from build123d import *

# Parameters (mm, degrees)
F0_W      = 1200
F0_H      = 2200
F1_DEPTH  = 40
F2_W      = 50
F2_H      = 1000
F3_DEPTH  = 10
F5_DEPTH  = 40.001
F6_R      = 25
F8_DEPTH  = 40.001
F9_W      = 25
F9_H      = 50
F10_DEPTH = 40.001
F12_D     = 14
F12_DEPTH = 31
F12_TIP   = 4.2060243332


with BuildPart() as f1:
    # F0 (on Front) → F1 (new body)
    with BuildSketch(Plane.XZ):
        Rectangle(F0_W, F0_H)
    extrude(amount=F1_DEPTH)

    # F2 (on face) → F3 (cut)
    with BuildSketch(Plane(origin=(0, 0, 0), x_dir=(-1, 0, 0), z_dir=(0, 1, 0))):
        with Locations((525, -600)):
            Rectangle(F2_W, F2_H)
    extrude(amount=-F3_DEPTH, mode=Mode.SUBTRACT)

    # F4 (on face) → F5 (cut, through all)
    with BuildSketch(Plane.XZ.offset(40)):
        with BuildLine():
            Line((-600, 300), (-600, 0))
            Line((-600, 0), (-350, 0))
            ThreePointArc((-350, 0), (-279.2893218813, 29.2893218813), (-250, 100))
            ThreePointArc((-250, 100), (-308.5786437627, 241.4213562373), (-450, 300))
            Line((-450, 300), (-600, 300))
        make_face()
    extrude(amount=-F5_DEPTH, mode=Mode.SUBTRACT)

    # F6
    f6_edges = [f1.edges().sort_by_distance(p)[0] for p in [
        (-600, -20, 300),
        (-600, -20, 0),
    ]]
    fillet(f6_edges, radius=F6_R)

    # F7 (on face) → F8 (cut, through all)
    with BuildSketch(Plane.XZ.offset(40)):
        with BuildLine():
            Line((-549.1, 1100), (-600, 1100))
            Line((-600, 1100), (-600, 325))
            ThreePointArc((-600, 325), (-592.6776695297, 307.3223304703), (-575, 300))
            Line((-575, 300), (-549.1, 300))
            Line((-549.1, 300), (-549.1, 1100))
        make_face()
    extrude(amount=-F8_DEPTH, mode=Mode.SUBTRACT)

    # F9 (on face) → F10 (cut, through all)
    with BuildSketch(Plane.XZ.offset(40)):
        with Locations((-587.5, -325)):
            Rectangle(F9_W, F9_H)
        with Locations((-587.5, -775)):
            Rectangle(F9_W, F9_H)
    extrude(amount=-F10_DEPTH, mode=Mode.SUBTRACT)

    # F12
    with Locations(Plane(origin=(-600, 0, 0), x_dir=(0, -1, 0), z_dir=(-1, 0, 0))):
        with Locations((20, -1050), (20, -950), (20, -850), (20, -700), (20, -600), (20, -500), (20, -400), (20, -250), (20, -150), (20, -50)):
            Hole(F12_D / 2, depth=F12_DEPTH)
            with Locations((0, 0, -(F12_DEPTH + F12_TIP / 2))):  # 118° drill point
                Cone(0, F12_D / 2, F12_TIP, mode=Mode.SUBTRACT)


solid = f1.part
Source: CAD feature listing. Evaluate the final solid. Frame: model axes, mm. A direction names the side the tool comes from. Give positions to 0.01 mm unless a question says otherwise; leave off trailing zeros. Loops run counter-clockwise (first coordinate to the right, second up) from the corner with the lowest first, then second, coordinate; pieces in that order, holes last. Notation, with made-up numbers: (67.5, 45) -> (96.5, 45) arc R27 cw to (96.5, 61) -> close; hole circle Ø8 at (24, -36.5). An arc over 180 degrees is marked (long way). Use a Markdown table: item, result. Add a question column.
1) Reachability of faces 4 (the face through (-464, -20, 0)), 5 (the face through (-8, -20, -1100)), 6 (the face through (-525, -10, -593)), 7 (the face through (-600, -20, -164)), 8 (the face through (-549.1, -20, 694)) from +Z, -Z, +X, -X, +Y, -Y: full face, straight path, thin tool, end or side. Return the list, or none.
2) Section query C-C, the plane z = 250. Return the cut outline in (x, y), then the cut area to 3 significant figures.
3) Section query B-B, the plane z = 588. Return the cut outline in (x, y).
4) Line query: line 1 along X through (y, z) = (-5, -876.5); line 2 along Y through (x, z) = (-581.5, -50); line 3 along X through (y, z) = (-3, 671). Output: solid intervals per line, ascending. Write a range as [from, to].
5) Pull-direction query (Z, two-part tool) for faces 1 (the face through (-600, -20, -553)), 2 (the face through (-575, -20, -325)), 3 (the face through (17, -20, 1100)); classes: +Z half, -Z half, draft (parallel to the pull), parting line (faces both ways), or undercut.
6) First-contact query: pin 1 (11 mm diameter, centred on y = -20, z = -700, fed in from -X); pin 2 (2 mm diameter, centred on y = -35, z = 664, fed in from -X); pin 3 (3 mm diameter, centred on x = -525, y = -5.5, fed in from -Z); pin 4 (18 mm diameter, centred on y = -20, z = -500, fed in from -X). Flat tips, straight axial feed; report the tip coordinate or a pass-through.
7) Section query A-A, the plane x = -321. Return the cut outline in (y, z).
Numbers:
| question | item | result |
|---|---|---|
| 1 | face 4 | -X, +Y, -Y |
| 1 | face 5 | -Z, +X, -X, +Y, -Y |
| 1 | face 6 | -Z, +Y |
| 1 | face 7 | +Z, -Z, -X, +Y, -Y |
| 1 | face 8 | +Z, -X, +Y, -Y |
| 2 | outline | (-317.71, -40) -> (600, -40) -> (600, 0) -> (-317.71, 0) -> close |
| 2 | area | 36,700 mm2 |
| 3 | outline | (-549.1, -40) -> (600, -40) -> (600, 0) -> (-549.1, 0) -> close |
| 4 | line 1 | x = [-600, -550], [-500, 600] |
| 4 | line 2 | y = [-40, -27], [-13, 0] |
| 4 | line 3 | x = [-549.1, 600] |
| 5 | face 1 | draft |
| 5 | face 2 | undercut |
| 5 | face 3 | +Z half |
| 6 | pin 1 | stops at x = -568.1 |
| 6 | pin 2 | stops at x = -549.1 |
| 6 | pin 3 | stops at z = -100 |
| 6 | pin 4 | stops at x = -600 |
| 7 | outline | (-40, -1100) -> (0, -1100) -> (0, 4.3) -> (-40, 4.3) -> close; (-40, 252.84) -> (0, 252.84) -> (0, 1100) -> (-40, 1100) -> close |
